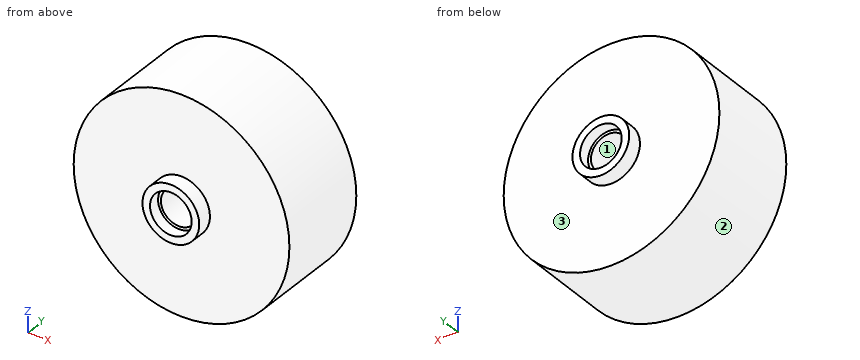
from build123d import *

# Parameters (mm, degrees)
EXTRUDE_1_DEPTH      = 12.5
EXTRUDE_1_DEPTH_BACK = 12.5
SKETCH_1_R           = 28.5
SKETCH_1_R_2         = 4.75
SKETCH_2_R           = 7.5
SKETCH_2_R_2         = 4.75
EXTRUDE_2_DEPTH      = 4
EXTRUDE_START        = 4
SKETCH_3_R           = 7.5
SKETCH_3_R_2         = 4.75
EXTRUDE_3_DEPTH      = 4
SKETCH_4_R           = 5.5
CUT_EXTRUDE_1_DEPTH  = 3
CUT_EXTRUDE_START    = -3
SKETCH_5_R           = 5.5
CUT_EXTRUDE_2_DEPTH  = 3


with BuildPart() as part:
    # 草图1 → 凸台-拉伸1 (new, two sides: drawn at the far end of the back side and taken through both)
    with BuildSketch(Plane(origin=(0, 0, 0), x_dir=(1, 0, 0), z_dir=(0, 1, 0)).offset(-EXTRUDE_1_DEPTH_BACK)):
        with Locations(Location((0, 0, 0), (0, 0, 270))):
            Circle(SKETCH_1_R)
        with Locations(Location((0, 0, 0), (0, 0, 270))):
            Circle(SKETCH_1_R_2, mode=Mode.SUBTRACT)
    extrude(amount=EXTRUDE_1_DEPTH + EXTRUDE_1_DEPTH_BACK)

    # 草图2 → 凸台-拉伸2 (add)
    with BuildSketch(Plane(origin=(0, 12.5, 0), x_dir=(1, 0, 0), z_dir=(0, 1, 0))):
        with Locations(Location((0, 0, 0), (0, 0, 270))):
            Circle(SKETCH_2_R)
        with Locations(Location((0, 0, 0), (0, 0, 270))):
            Circle(SKETCH_2_R_2, mode=Mode.SUBTRACT)
    extrude(amount=EXTRUDE_2_DEPTH)

    # 草图3 → 凸台-拉伸3 (add)
    with BuildSketch(Plane(origin=(0, -12.5, 0), x_dir=(-1, 0, 0), z_dir=(0, -1, 0)).offset(EXTRUDE_START)):
        with Locations(Location((0, 0, 0), (0, 0, 270))):
            Circle(SKETCH_3_R)
        with Locations(Location((0, 0, 0), (0, 0, 270))):
            Circle(SKETCH_3_R_2, mode=Mode.SUBTRACT)
    extrude(amount=-EXTRUDE_3_DEPTH)

    # 草图4 → 切除-拉伸1 (cut)
    with BuildSketch(Plane(origin=(0, 16.5, 0), x_dir=(1, 0, 0), z_dir=(0, 1, 0))):
        with Locations(Location((0, 0, 0), (0, 0, 270))):
            Circle(SKETCH_4_R)
    extrude(amount=-CUT_EXTRUDE_1_DEPTH, mode=Mode.SUBTRACT)

    # 草图5 → 切除-拉伸2 (cut)
    with BuildSketch(Plane(origin=(0, -16.5, 0), x_dir=(-1, 0, 0), z_dir=(0, -1, 0)).offset(CUT_EXTRUDE_START)):
        with Locations(Location((0, 0, 0), (0, 0, 270))):
            Circle(SKETCH_5_R)
    extrude(amount=CUT_EXTRUDE_2_DEPTH, mode=Mode.SUBTRACT)


solid = part.part
Source: CAD feature listing. Evaluate the final solid. Frame: model axes, mm. Face numbers are marked on the shaded views. Give positions to 0.01 mm unless a question says otherwise; leave off trailing zeros. Write each loop counter-clockwise with the first axis right and the second up, starting at its lowest first coordinate (ties: lowest second). Pieces come first, ordered by that corner, then holes. Notation, with made-up numbers: M 61.5,-33 L 96.5,-33 A15 cw 96.5,-7 Z; hole C -21,33 d4. An arc over 180 degrees is marked long. Return JSON: item names as keys, results as strings. Group by question number.
1) Cut plane D-D, the plane z = -16. Output: boundary loops of the cut face in (x, y).
2) Cut plane A-A, the plane x = 0. Output: boundary loops of the cut face in (y, z), plus the area to 3 significant figures.
3) Pull-direction query (X, two-part tool) for the marked faces 1, 2 and 3; classes: pulls with the +X half, pulls with the -X half, needs draft (parallel to the pull), parting line crosses it, or undercut.
4) Pin query (flat end, axial travel): P1, Ø10, axis at y = -3.5, z = -14.5, coming from the +X side; P2, Ø5, axis at x = 19, z = -8.5, coming from the +Y side; P3, Ø4, axis at y = 7.5, z = 11, coming from the +X side. Return the tip coordinate at first contact, or that it passes through.
5) Material intervals for line 1 along X through (y, z) = (-1, 0); line 2 along X through (y, z) = (15.35, 0); line 3 along Y through (x, z) = (17.5, 1.5), sorted ascending. Write a range as [from, to].
6) Cut plane B-B, the plane z = 0. Output: boundary loops of the cut face in (x, y).
7) Cut plane C-C, the plane y = 7. Output: boundary loops of the cut face in (x, z), plus the area to 3 significant figures.
Recorded:
{
 "1": {"outline": "M -23.58,-12.5 L 23.58,-12.5 L 23.58,12.5 L -23.58,12.5 Z"},
 "2": {"outline": "M -16.5,-7.5 L -12.5,-7.5 L -12.5,-28.5 L 12.5,-28.5 L 12.5,-7.5 L 16.5,-7.5 L 16.5,-5.5 L 13.5,-5.5 L 13.5,-4.75 L -13.5,-4.75 L -13.5,-5.5 L -16.5,-5.5 Z; M -16.5,5.5 L -13.5,5.5 L -13.5,4.75 L 13.5,4.75 L 13.5,5.5 L 16.5,5.5 L 16.5,7.5 L 12.5,7.5 L 12.5,28.5 L -12.5,28.5 L -12.5,7.5 L -16.5,7.5 Z", "area": "1,220 mm²"},
 "3": {"face 1": "undercut", "face 2": "parting line crosses it", "face 3": "needs draft"},
 "4": {"P1": "stops at x = 26.87", "P2": "stops at y = 12.5", "P3": "stops at x = 27.04"},
 "5": {"line 1": "x = [-28.5, -4.75], [4.75, 28.5]", "line 2": "x = [-7.5, -5.5], [5.5, 7.5]", "line 3": "y = [-12.5, 12.5]"},
 "6": {"outline": "M -28.5,-12.5 L -7.5,-12.5 L -7.5,-16.5 L -5.5,-16.5 L -5.5,-13.5 L -4.75,-13.5 L -4.75,13.5 L -5.5,13.5 L -5.5,16.5 L -7.5,16.5 L -7.5,12.5 L -28.5,12.5 Z; M 4.75,-13.5 L 5.5,-13.5 L 5.5,-16.5 L 7.5,-16.5 L 7.5,-12.5 L 28.5,-12.5 L 28.5,12.5 L 7.5,12.5 L 7.5,16.5 L 5.5,16.5 L 5.5,13.5 L 4.75,13.5 Z"},
 "7": {"outline": "C 0,0 d57; hole C 0,0 d9.5", "area": "2,480 mm²"}
}
